Read the model definition and answer for the solid it produces. Units are mm, in the model's axes. Coordinates: 2 decimals unless noted, no trailing zeros. Order: outer loops, then holes, each group sorted by start corner. A loop starts at its lowest first (then second) coordinate and runs counter-clockwise, first axis right, second up.
Autodesk Inventor part; units mm, degrees
ref_plane "YZ Plane" through (0, 0, 0) normal (1, 0, 0) x (0, 1, 0)
ref_plane "XZ Plane" through (0, 0, 0) normal (0, 1, 0) x (-1, 0, 0)
ref_plane "XY Plane" through (0, 0, 0) normal (0, 0, 1) x (1, 0, 0)
sketch "Sketch1" plane through (0, 0, 0) normal (0, 0, 1) x (1, 0, 0)
  line L0 (-83.8471, 83.8315) -> (93.9529, 83.8315)
  line L1 (93.9529, 83.8315) -> (93.9529, 20.3315)
  line L2 (93.9529, 20.3315) -> (-83.8471, 20.3315)
  line L3 (-83.8471, 20.3315) -> (-83.8471, 83.8315)
  line L4 (-83.8471, 20.3315) -> (-83.8471, 58.4315)
  line L5 (93.9529, 20.3315) -> (93.9529, 58.2798)
  line L6 (93.9529, 58.2798) -> (60.1807, 20.3315)
  line L7 (-83.8471, 58.4315) -> (-50.246, 20.3315)
  circle A0 centre (-58.4471, 77.4815) radius 2.54
  circle A1 centre (68.5529, 77.4815) radius 2.54
  circle A2 centre (2.5129, 26.6815) radius 2.54
  circle A3 centre (-45.7471, 26.6815) radius 2.54
  circle A4 centre (55.8529, 26.6815) radius 2.54
  line L8 (-58.4471, 77.4815) -> (-71.1471, 77.4815)
  circle A5 centre (-71.1471, 77.4815) radius 2.54
  line L9 (-71.1471, 77.4815) -> (-71.1471, 64.7815)
  line L10 (-71.1471, 64.7815) -> (-58.4471, 64.7815)
  circle A6 centre (-71.1471, 64.7815) radius 2.54
  circle A7 centre (-58.4471, 64.7815) radius 2.54
  line L11 (-58.4471, 77.4815) -> (5.0529, 77.4815)
  line L12 (5.0529, 77.4815) -> (-7.6471, 77.4815)
  circle A8 centre (-7.6471, 77.4815) radius 2.54
  circle A9 centre (5.0529, 77.4815) radius 2.54
  line L13 (5.0529, 77.4815) -> (17.7529, 77.4815)
  circle A10 centre (17.7529, 77.4815) radius 2.54
  line L14 (68.5529, 77.4815) -> (81.2529, 77.4815)
  line L15 (81.2529, 77.4815) -> (81.2529, 64.7815)
  line L16 (81.2529, 64.7815) -> (68.5529, 64.7815)
  circle A11 centre (81.2529, 77.4815) radius 2.54
  circle A12 centre (81.2529, 64.7815) radius 2.54
  circle A13 centre (68.5529, 64.7815) radius 2.54
  point P0 (0, 0)
  dimension "d0" = 177.8
  dimension "d1" = 63.5
  dimension "d2" = 38.1
  dimension "d3" = 50.8
  dimension "d4" = 50.8
  dimension "d18" = 6.35
  dimension "d19" = 25.4
  dimension "d20" = 5.08
  dimension "d21" = 5.08
  dimension "d22" = 6.35
  dimension "d23" = 25.4
  dimension "d24" = 5.08
  dimension "d25" = 6.35
  dimension "d26" = 86.36
  dimension "d29" = 6.35
  dimension "d30" = 6.35
  dimension "d31" = 38.1
  dimension "d32" = 38.1
  dimension "d33" = 5.08
  dimension "d34" = 5.08
  dimension "d39" = 12.7
  dimension "d40" = 5.08
  dimension "d41" = 12.7
  dimension "d42" = 5.08
  dimension "d43" = 5.08
  dimension "d44" = 12.7
  dimension "d45" = 5.08
  dimension "d46" = 5.08
  dimension "d47" = 12.7
  dimension "d48" = 5.08
  dimension "d49" = 12.7
  dimension "d50" = 12.7
  dimension "d51" = 12.7
  dimension "d52" = 5.08
  dimension "d53" = 5.08
  dimension "d54" = 5.08
extrude "Extrusion3" add sketch "Sketch1" along normal blind 1.5875 contours L0 L1 L6 L2 L7 L3
fillet "Fillet6" radius 3.175 4 edges at (-83.8471, 58.4315, 0.7937) (-50.246, 20.3315, 0.7937) (60.1807, 20.3315, 0.7937) (-83.8471, 83.8315, 0.7937)
fillet "Fillet7" radius 3.175 2 edges at (93.9529, 83.8315, 0.7937) (93.9529, 58.2798, 0.7937)
properties part number "wedge"
1) Straight lines are drawn through the part: line 1 (X direction, y = 64.5, z = 0.15); line 2 (X direction, y = 63, z = 0.95); line 3 (Y direction, x = -6, z = 0.55). For each, find the intervals that lie inside material, in ascending order.
A:
line 1: x = -83.85 to -73.67, -68.62 to -60.97, -55.92 to 66.03, 71.08 to 78.73, 83.78 to 93.95
line 2: x = -83.85 to -72.96, -69.34 to -60.26, -56.64 to 66.74, 70.36 to 79.44, 83.06 to 93.95
line 3: y = 20.33 to 75.55, 79.42 to 83.83
2) A cutting plane is placed at D-D, the plane y = 51.5. Determine the outline of the cut face in (x, z), and give its area (3 significant figures).
A:
outline: (-77.73, 0) - (87.92, 0) - (87.92, 1.59) - (-77.73, 1.59) - close
area: 263 mm2
3) A cutting plane is placed at B-B, the plane z = 1.3. State how many separate pieces and enclosed holes the cut face has, and give its area (3 significant figures).
A:
separate pieces: 1
enclosed holes: 14
area: 9,720 mm2
4) A cutting plane is placed at C-C, the plane y = 34. Determine the outline of the cut face in (x, z), and give its area (3 significant figures).
A:
outline: (-62.3, 0) - (72.35, 0) - (72.35, 1.59) - (-62.3, 1.59) - close
area: 214 mm2
5) A cutting plane is placed at A-A, the plane x = -71.5. Determine the outline of the cut face in (y, z), and give its area (3 significant figures).
A:
outline: (44.43, 0) - (62.27, 0) - (62.27, 1.59) - (44.43, 1.59) - close; (67.3, 0) - (74.97, 0) - (74.97, 1.59) - (67.3, 1.59) - close; (80, 0) - (83.83, 0) - (83.83, 1.59) - (80, 1.59) - close
area: 46.6 mm2
6) Determine the mould class of faces 1 (the flat face through (4, 53, 0)), 2 (the flat face through (-67.347, 39.722, 0.783)), 3 (the cylindrical face through (-7.978, 74.963, 0.783)) for opening direction X: pulls with the +X half, pulls with the -X half, needs draft (parallel to the pull), parting line crosses it, or undercut.
A:
face 1: needs draft
face 2: pulls with the -X half
face 3: undercut
